Geometry: final body of the model. Coordinates: model frame, mm. A direction names the side the tool comes from. Coordinates: 2 decimals unless noted, no trailing zeros. Order: outer loops, then holes, each group sorted by start corner. A loop starts at its lowest first (then second) coordinate and runs counter-clockwise, first axis right, second up. Notation, with made-up numbers: (5.5, -9) -> (37.5, -9) arc R26 ccw to (37.5, 27) -> close; hole circle Ø7 at (68.5, 29). An arc over 180 degrees is marked (long way). Use CSV: the item, a comma, the result in double quotes. Start each with the question number.
Autodesk Inventor part; units mm, degrees
ref_plane "YZ Plane" through (0, 0, 0) normal (1, 0, 0) x (0, 1, 0)
ref_plane "XZ Plane" through (0, 0, 0) normal (0, 1, 0) x (-1, 0, 0)
ref_plane "XY Plane" through (0, 0, 0) normal (0, 0, 1) x (1, 0, 0)
sketch "Esboço1" plane through (0, 0, 0) normal (0, 1, 0) x (-1, 0, 0)
  arc A0 (-410, 0) -> (-289.9138, -289.9138) centre (0, 0) ccw
  arc A1 (-460, 0) -> (-325.2691, -325.2691) centre (0, 0) ccw
  circle A2 centre (0, 0) radius 460
  circle A3 centre (0, 0) radius 410
  line L0 (0, 0) -> (-407.9373, -407.9373)
  line L1 (0, 0) -> (-1224.3013, 0) construction
  line L2 (-410, 0) -> (-460, 0)
  point P0 (-460, 0)
  point P1 (-325.2691, -325.2691)
  point P2 (-289.9138, -289.9138)
  dimension "d27" = 820
  dimension "d28" = 920
  dimension "d87" = 45
extrude "Extrusão1" add sketch "Esboço1" along normal blind 6 contours A0 L0 A1 L2
sketch "Esboço6" plane through (0, 6, 0) normal (0, 1, 0) x (1, 0, 0)
  arc A0 (460, 0) -> (325.2691, 325.2691) centre (0, 0) ccw
  circle A1 centre (0, 0) radius 460
  arc A2 (410, 0) -> (289.9138, 289.9138) centre (0, 0) ccw
  circle A3 centre (0, 0) radius 410
  line L0 (0, 0) -> (743.005, 65.0045)
  line L1 (410, 0) -> (460, 0)
  line L2 (410, 0) -> (428, 0)
  line L3 (428, 0) -> (442, 0)
  line L4 (408.4398, 35.7339) -> (423.3827, 37.0412)
  line L5 (423.3827, 37.0412) -> (443.3066, 38.7843)
  line L6 (428, 0) -> (423.3827, 37.0412)
  line L7 (442, 0) -> (443.3066, 38.7843)
  dimension "d110" = -5
  dimension "d111" = 18
  dimension "d112" = 14
  dimension "d113" = 15
  dimension "d114" = 20
extrude "Extrusão6" cut sketch "Esboço6" against normal up to surface (6 mm away) contours L1 L6 L0 L7
sketch "Esboço8" plane through (0, 6, 0) normal (0, 1, 0) x (1, 0, 0)
  arc A0 (325.2691, 325.2691) -> (352.3804, 295.6823) centre (0, 0) ccw
  arc A1 (289.9138, 289.9138) -> (314.0782, 263.5429) centre (0, 0) ccw
  line L0 (0, 0) -> (489.696, 410.9037)
  line L1 (325.2691, 325.2691) -> (289.9138, 289.9138)
  line L2 (325.2691, 325.2691) -> (314.6625, 314.6625)
  line L3 (314.6625, 314.6625) -> (300.5204, 300.5204)
  line L4 (352.3804, 295.6823) -> (338.5916, 284.1121)
  line L5 (338.5916, 284.1121) -> (327.867, 275.1131)
  line L6 (327.867, 275.1131) -> (300.5204, 300.5204)
  line L7 (338.5916, 284.1121) -> (314.6625, 314.6625)
  circle A2 centre (0, 0) radius 460
  circle A3 centre (0, 0) radius 410
  point P0 (314.0782, 263.5429)
  point P1 (352.3804, 295.6823)
  point P2 (325.2691, 325.2691)
  dimension "d130" = -5
  dimension "d131" = 15
  dimension "d132" = 20
  dimension "d133" = 18
  dimension "d134" = 14
extrude "Extrusão7" cut sketch "Esboço8" against normal up to surface (6 mm away) contours A2 L0 L7 L1 | L6 L0 A3 L1
equation "\"Raio_vergadura\" = Espessura"
equation "\"Largura_alívio_de_vergadura\" = Espessura"
equation "\"Profundidade_alívio_de_vergadura\" = 0.5 * Espessura"
equation "\"Tamanho_alívio_de_dobra\" = 4 * Espessura"
equation "\"Remanescente_mínimo\" = 2 * Espessura"
equation "\"Raiodetransição\" = Raio_vergadura"
equation "\"Tamanho_de_raio_de_Jacobi\" = Raio_vergadura"
equation "\"TamanhoFolga\" = Espessura"
properties part number "base"
(1) Section C-C (z = -86.5). Return loops of the section in (x, y).
(2) First-contact query: pin 1 (1 mm diameter, centred on x = 389, y = 1, fed in from -Z); pin 2 (1 mm diameter, centred on x = 416, y = 5, fed in from -Z); pin 3 (2 mm diameter, centred on x = 422.5, y = 1.5, fed in from -Z). Flat tips, straight axial feed; report the tip coordinate or a pass-through.
(3) Access query for faces 1 (the face through (433.2, 3, -37.9)), 2 (the face through (320.88, 3.04, -269.25)), 3 (the face through (345.39, 3.042, -289.816)), 4 (the face through (398, 6, -157)). Directions: +Z, -Z, +X, -X, +Y, -Y. A direction counts if a zero-diameter tool reaches every point of the face in a straight line with its end or side. Return the directions, or none.
(4) Section A-A (x = 323). Return loops of the section in (y, z).
(5) Section B-B (y = 1.5). Return loops of the section in (x, z), then the cut area to 3 significant figures.
(6) Line query: line 1 (X direction, y = 5.4, z = -14); line 2 (X direction, y = 3.35, z = -22.5); line 3 (X direction, y = 2.8, z = -184). Output: solid intervals per line, ascending. Write a range as from..to.
(7) Mould query, pull axis X, two halves, no side actions, for faces 5 (the face through (314.385, 3.042, -287.639)), 6 (the face through (451, 3, 0)), 7 (the face through (326.795, 3.042, -299.173)). Classes: pulls with the +X half, pulls with the -X half, needs draft (parallel to the pull), parting line crosses it, or undercut.
(8) Section D-D (x = 448.5). Return loops of the section in (y, z), then the cut area to 3 significant figures.
Check sheet entries:
1,outline,"(400.77, 0) -> (451.79, 0) -> (451.79, 6) -> (400.77, 6) -> close"
2,pin 1,"stops at z = -246.31"
2,pin 2,"stops at z = -197.38"
2,pin 3,"stops at z = -184.22"
3,face 1,"+Y, -Y"
3,face 2,"-X, +Y, -Y"
3,face 3,"-Z, +Y, -Y"
3,face 4,"+Z, -Z, +X, -X, +Y"
4,outline,"(0, -304.02) -> (6, -304.02) -> (6, -279.63) -> (0, -279.63) -> close; (0, -271.03) -> (6, -271.03) -> (6, -252.53) -> (0, -252.53) -> close"
5,outline,"(300.52, -300.52) -> (314.66, -314.66) -> (338.59, -284.11) -> (352.38, -295.68) arc R460 ccw to (460, 0) -> (442, 0) -> (443.31, -38.78) -> (423.38, -37.04) -> (428, 0) -> (410, 0) arc R410 cw to (314.08, -263.54) -> (327.87, -275.11) -> close"
5,area,"15,200 mm^2"
6,line 1,"x = 409.76..426.25, 442.47..459.79"
6,line 2,"x = 409.38..425.2, 442.76..459.45"
6,line 3,"x = 366.39..421.6"
7,face 5,"pulls with the -X half"
7,face 6,"needs draft"
7,face 7,"undercut"
8,outline,"(0, -102.21) -> (6, -102.21) -> (6, 0) -> (0, 0) -> close"
8,area,"613 mm^2"
